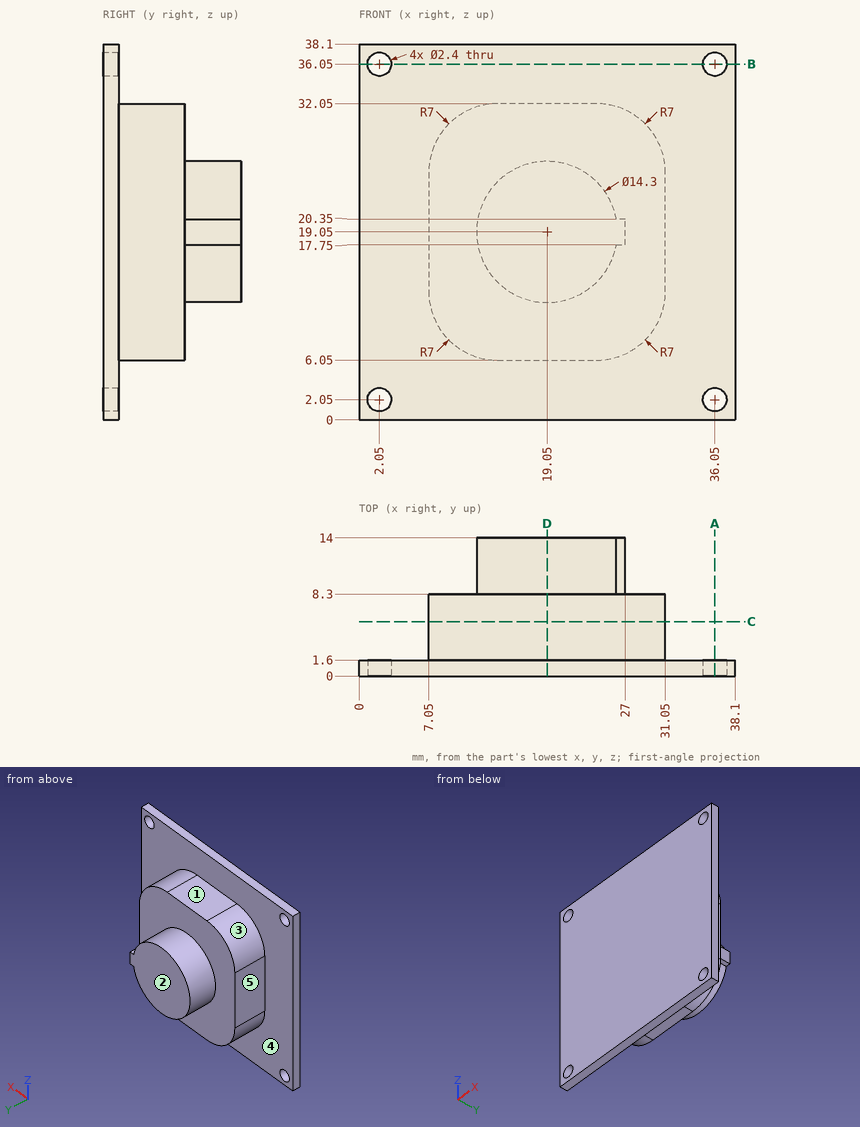
Source: three-view drawing plus pictorial views. Frame: mm from the lowest corner of the part. A direction names the side the tool comes from. Give positions to 0.01 mm unless a question says otherwise; leave off trailing zeros. Write each loop counter-clockwise with the first axis right and the second up, starting at its lowest first coordinate (ties: lowest second). Pieces come first, ordered by that corner, then holes. Notation, with made-up numbers: (-5, 53) -> (50, 53) arc R22 ccw to (50, 68) -> close; hole circle Ø5 at (26, 12). An arc over 180 degrees is marked (long way). Write item = value, one per line.
Q1. Reachability of the marked faces 1, 2, 3, 4 and 5 from +Z, -Z, +X, -X, +Y, -Y: full face, straight path, thin tool, end or side. Return the list, or none.
Here are the results:
face_1 = +Z, +X, -X, +Y
face_2 = +Z, -Z, +X, -X, +Y
face_3 = +Z, -X, +Y
face_4 = +Y
face_5 = +Z, -Z, -X, +Y
Q2. Cut plane B-B on z = 36.05. Return loops of the section in (x, y).
Here are the results:
outline = (0, 0) -> (0.85, 0) -> (0.85, 1.6) -> (0, 1.6) -> close; (3.25, 0) -> (34.85, 0) -> (34.85, 1.6) -> (3.25, 1.6) -> close; (37.25, 0) -> (38.1, 0) -> (38.1, 1.6) -> (37.25, 1.6) -> close
Q3. First-contact query: pin 1 (2 mm diameter, centred on y = 3.5, z = 19.5, fed in from -X); pin 2 (3 mm diameter, centred on y = 8.5, z = 8.5, fed in from +X); pin 3 (6 mm diameter, centred on y = 12.5, z = 12.5, fed in from +X). Flat tips, straight axial feed; report the tip coordinate or a pass-through.
Here are the results:
pin_1 = 7.05
pin_2 = 30.34
pin_3 = 25.26
Q4. Cut plane C-C on y = 5.5. Return loops of the section in (x, z).
Here are the results:
outline = (7.05, 13.05) arc R7 ccw to (14.05, 6.05) -> (24.05, 6.05) arc R7 ccw to (31.05, 13.05) -> (31.05, 25.05) arc R7 ccw to (24.05, 32.05) -> (14.05, 32.05) arc R7 ccw to (7.05, 25.05) -> close
Q5. Cut plane D-D on x = 19.05. Return loops of the section in (y, z).
Here are the results:
outline = (0, 0) -> (1.6, 0) -> (1.6, 6.05) -> (8.3, 6.05) -> (8.3, 11.9) -> (14, 11.9) -> (14, 26.2) -> (8.3, 26.2) -> (8.3, 32.05) -> (1.6, 32.05) -> (1.6, 38.1) -> (0, 38.1) -> close
Q6. Line query: line 1 (X direction, y = 0.9, z = 36.05); line 2 (Y direction, x = 36, z = 29); line 3 (Z direction, x = 23.5, y = 7.25). Output: solid intervals per line, ascending. Write a range as from..to.
Here are the results:
line_1 = 0..0.85, 3.25..34.85, 37.25..38.1
line_2 = 0..1.6
line_3 = 6.05..32.05
Q7. Cut plane A-A on x = 36.05. Return loops of the section in (y, z).
Here are the results:
outline = (0, 0) -> (1.6, 0) -> (1.6, 0.85) -> (0, 0.85) -> close; (0, 3.25) -> (1.6, 3.25) -> (1.6, 34.85) -> (0, 34.85) -> close; (0, 37.25) -> (1.6, 37.25) -> (1.6, 38.1) -> (0, 38.1) -> close
